Check sheet for the drawn part. Datum: minimum x, y, z corner. Units: mm. A direction names the side the tool comes from. Round coordinates to 2 decimals unless told otherwise and drop trailing zeros. Write each loop counter-clockwise with the first axis right and the second up, starting at its lowest first coordinate (ties: lowest second). Pieces come first, ordered by that corner, then holes. Notation, with made-up numbers: (18, 79.25) -> (62, 79.25) arc R18 cw to (62, 110.25) -> close; hole circle Ø3 at (17, 50). An arc over 180 degrees is marked (long way). Use a Markdown table: item, result.
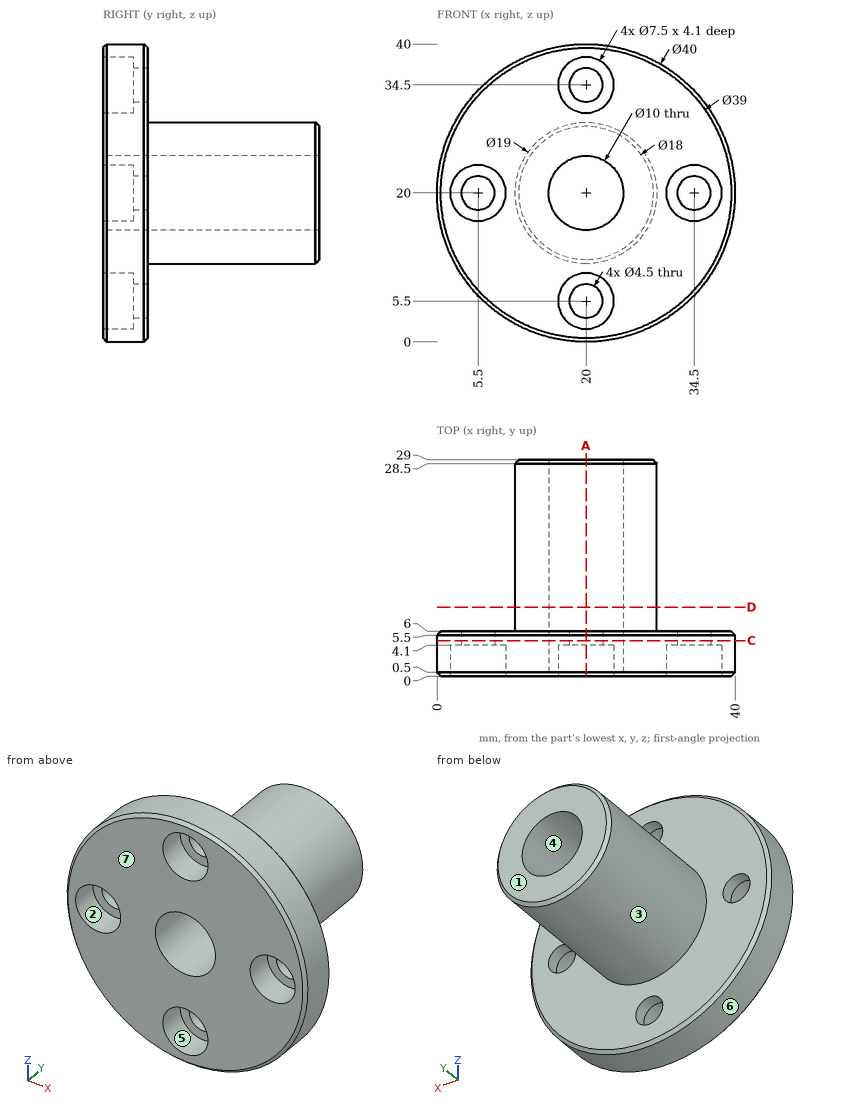
(1) Section check C-C on y = 4.75. Record the cut outline in (x, z).
A:
| item | result |
|---|---|
| outline | circle Ø40 at (20, 20); hole circle Ø4.5 at (5.5, 20); hole circle Ø10 at (20, 20); hole circle Ø4.5 at (20, 5.5); hole circle Ø4.5 at (20, 34.5); hole circle Ø4.5 at (34.5, 20) |
(2) Section check A-A on x = 20. State how many separate pieces and enclosed holes the cut face has, plus the area to 3 significant figures.
A:
| item | result |
|---|---|
| separate pieces | 4 |
| enclosed holes | 0 |
| area | 308 mm2 |
(3) Release check for a two-part mould opening along Z. For the marked faces 4, 5, 6 and 7 record: +Z half, -Z half, draft (parallel to the pull), parting line (faces both ways), or undercut.
A:
| item | result |
|---|---|
| face 4 | undercut |
| face 5 | undercut |
| face 6 | parting line |
| face 7 | draft |
(4) Thickness scan on line 1 (X direction, y = 5.25, z = 20); line 2 (X direction, y = 8, z = 20); line 3 (Y direction, x = 18.5, z = 3.5). Record the ranges inside material, lowest first.
A:
| item | result |
|---|---|
| line 1 | x = 0 to 3.25, 7.75 to 15, 25 to 32.25, 36.75 to 40 |
| line 2 | x = 10.5 to 15, 25 to 29.5 |
| line 3 | y = 4.1 to 6 |
(5) Gauge pin test, flat ends, axial feed: pin 1 Ø8.5 at (x, z) = (34.5, 20) entering from +Y; pin 2 Ø4 at (x, z) = (19, 5.5) entering from -Y; pin 3 Ø4 at (x, y) = (18.5, 10) entering from -Z; pin 4 Ø2.5 at (x, z) = (20, 5.5) entering from +Y. Record the tip position at first contact, or that the pin passes through.
A:
| item | result |
|---|---|
| pin 1 | stops at y = 6 |
| pin 2 | stops at y = 4.1 |
| pin 3 | stops at z = 10.5 |
| pin 4 | passes through |
(6) Section check D-D on y = 9.25. Record the cut outline in (x, z).
A:
| item | result |
|---|---|
| outline | circle Ø19 at (20, 20); hole circle Ø10 at (20, 20) |
(7) Access from +Z, -Z, +X, -X, +Y, -Y to the whole of each face (thin tool, end or side, straight path). Record for the marked faces 1, 2 and 3.
A:
| item | result |
|---|---|
| face 1 | +Z, -Z, +X, -X, +Y |
| face 2 | -Y |
| face 3 | +Y |
